Part model, mm, in its own coordinate system. Face numbers are marked on the shaded views. A direction names the side the tool comes from. Round coordinates to 2 decimals unless told otherwise and drop trailing zeros. Loops run counter-clockwise (first coordinate to the right, second up) from the corner with the lowest first, then second, coordinate; pieces in that order, holes last. Notation, with made-up numbers: (26, -37.75) -> (69, -37.75) arc R14 cw to (69, -12.75) -> close; hole circle Ø8 at (20, 32.25). An arc over 180 degrees is marked (long way). Use a Markdown table: item, result. Add a question column.
Item 1: Which spindle directions (+Z, -Z, +X, -X, +Y, -Y) get a long thin tool onto all of the face, cutting with end or side? Do the marked faces 1 and 2. Say none if no direction does.
Item 2: Two-plate mould, pull along Z, no slides. Class the marked faces 3, 4, 5 and 6: pulls with the +Z half, pulls with the -Z half, needs draft (parallel to the pull), parting line crosses it, or undercut.
Item 3: Flat gauge pins, fed straight in: pin 1 (1.5 mm diameter, centred on x = -13.5, z = 5.5, fed in from +Y); pin 2 (1 mm diameter, centred on x = -23, z = 5.5, fed in from -Y); pin 3 (12 mm diameter, centred on x = 11.5, z = 15.5, fed in from -Y). Where does each tip first touch, or does it go through?
Item 4: Cut at A-A, the plane y = -86. List the corners of the cut face in (x, z).
Item 5: Probe line 1 (Z direction, x = 33, y = -60); line 2 (Y direction, x = 24.5, z = 2.25); line 3 (X direction, y = -83, z = 11). List the from-to ranges inside material, lowest first. Write a range as [from, to].
Item 6: Cut at B-B, the plane z = 9.25. List the corners of the cut face in (x, y).
```python
from build123d import *

# Parameters (mm, degrees)
SKETCH_1_R          = 42.2
SKETCH_1_R_2        = 41
EXTRUDE_1_DEPTH     = 21
SKETCH_2_R          = 51.055310859
SKETCH_2_R_2        = 42.2
EXTRUDE_2_DEPTH     = 3
SKETCH_3_R          = 1.5
CUT_EXTRUDE_1_DEPTH = 12
EXTRUDE1_START      = -3
SKETCH1_R           = 51.055310859
SKETCH1_R_2         = 42.2
SKETCH1_R_3         = 1.6
EXTRUDE1_DEPTH      = 3
CHAMFER1_SIZE       = 1


with BuildPart() as part:
    # 草图1 → 凸台-拉伸1 (new body)
    with BuildSketch(Plane.XY):
        with Locations((-1.800213466, -86)):
            Circle(SKETCH_1_R)
        with Locations((-1.800213466, -86)):
            Circle(SKETCH_1_R_2, mode=Mode.SUBTRACT)
    extrude(amount=EXTRUDE_1_DEPTH)

    # 草图2 → 凸台-拉伸2 (add)
    with BuildSketch(Plane(origin=(0, 0, 0), x_dir=(-1, 0, 0), z_dir=(0, 0, -1))):
        with Locations((1.800213466, -86)):
            Circle(SKETCH_2_R)
        with Locations((1.800213466, -86)):
            Circle(SKETCH_2_R_2, mode=Mode.SUBTRACT)
    extrude(amount=-EXTRUDE_2_DEPTH)

    # 草图3 → 切除-拉伸1 (cut)
    with BuildSketch(Plane.XY.offset(3)):
        with Locations((44.771512493, -95.028924631)):
            Circle(SKETCH_3_R)
        with Locations((-2.651398789, -38.568759005)):
            Circle(SKETCH_3_R)
        with Locations((41.858407753, -67.4427391)):
            Circle(SKETCH_3_R)
        with Locations((24.017335287, -46.20174231)):
            Circle(SKETCH_3_R)
        with Locations((-46.096553953, -69.021149678)):
            Circle(SKETCH_3_R)
        with Locations((-29.029091447, -47.153695895)):
            Circle(SKETCH_3_R)
    extrude(amount=-CUT_EXTRUDE_1_DEPTH, mode=Mode.SUBTRACT)

    # Sketch1 → Extrude1 (add)
    with BuildSketch(Plane.XY.offset(21).offset(EXTRUDE1_START)):
        with Locations(Location((-1.800213466, -86, 0), (0, 0, 180))):
            Circle(SKETCH1_R)
        with Locations(Location((-1.800213466, -86, 0), (0, 0, 180))):
            Circle(SKETCH1_R_2, mode=Mode.SUBTRACT)
        with Locations((-25.050213466, -45.729818724)):
            Circle(SKETCH1_R_3, mode=Mode.SUBTRACT)
        with Locations((21.449786534, -45.729818724)):
            Circle(SKETCH1_R_3, mode=Mode.SUBTRACT)
        with Locations((44.699786534, -86)):
            Circle(SKETCH1_R_3, mode=Mode.SUBTRACT)
        with Locations((21.449786534, -126.270181276)):
            Circle(SKETCH1_R_3, mode=Mode.SUBTRACT)
        with Locations((-25.050213466, -126.270181276)):
            Circle(SKETCH1_R_3, mode=Mode.SUBTRACT)
        with Locations((-48.300213466, -86)):
            Circle(SKETCH1_R_3, mode=Mode.SUBTRACT)
    extrude(amount=EXTRUDE1_DEPTH)

    # Chamfer1
    chamfer1_edges = [part.edges().sort_by_distance(p)[0] for p in [
        (-44.000213466, -86, 3),
        (-44.000213466, -86, 18),
    ]]
    chamfer(chamfer1_edges, length=CHAMFER1_SIZE)


solid = part.part
```
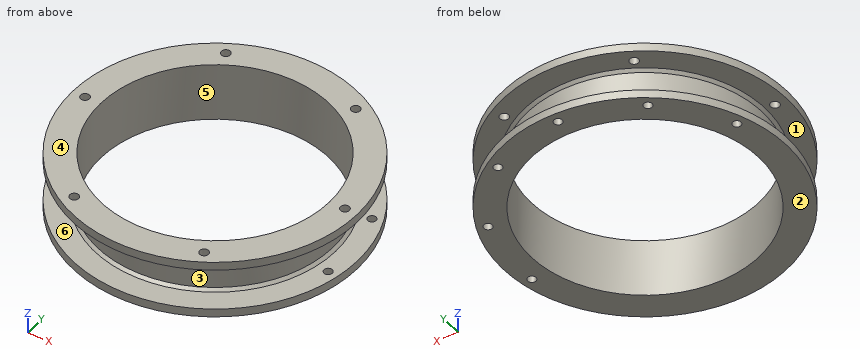
A:
| question | item | result |
|---|---|---|
| 1 | face 1 | none |
| 1 | face 2 | -Z, +X, -X, +Y, -Y |
| 2 | face 3 | undercut |
| 2 | face 4 | pulls with the +Z half |
| 2 | face 5 | needs draft |
| 2 | face 6 | undercut |
| 3 | pin 1 | stops at y = -45.25 |
| 3 | pin 2 | stops at y = -122.77 |
| 3 | pin 3 | stops at y = -136.45 |
| 4 | outline | (-52.86, 0) -> (-42.8, 0) -> (-42.8, 21) -> (-46.7, 21) -> (-46.7, 18) -> (-45, 18) -> (-44, 17) -> (-44, 4) -> (-45, 3) -> (-52.86, 3) -> close; (-52.86, 18) -> (-49.9, 18) -> (-49.9, 21) -> (-52.86, 21) -> close; (39.2, 0) -> (49.26, 0) -> (49.26, 3) -> (41.4, 3) -> (40.4, 4) -> (40.4, 17) -> (41.4, 18) -> (43.1, 18) -> (43.1, 21) -> (39.2, 21) -> close; (46.3, 18) -> (49.26, 18) -> (49.26, 21) -> (46.3, 21) -> close |
| 5 | line 1 | z = [0, 3], [18, 21] |
| 5 | line 2 | y = [-129.76, -117.45], [-54.55, -47.62], [-44.78, -42.24] |
| 5 | line 3 | x = [-43.89, -42.69], [39.09, 40.29] |
| 6 | outline | circle Ø84.4 at (-1.8, -86); hole circle Ø82 at (-1.8, -86) |
